The listing builds one solid part. Answer for the finished solid, in the listing's coordinates (mm). A direction names the side the tool comes from. Coordinates: 2 decimals unless noted, no trailing zeros. Loops run counter-clockwise (first coordinate to the right, second up) from the corner with the lowest first, then second, coordinate; pieces in that order, holes last. Notation, with made-up numbers: M 12,-7 L 57,-7 A13 cw 57,4 Z; hole C 51.5,86.5 d1. An arc over 180 degrees is marked long. Answer as a JSON object with one key per item and string values. Group by question number.
1. A cutting plane is placed at A-A on z = 5. Give the vertices of the cut face in (x, y).
2. A cutting plane is placed at C-C on y = 19.75. Give the vertices of the cut face in (x, z), and give its area (3 significant figures).
3. Given pin 1 (10 mm diameter, centred on x = -7, y = 18.5, fed in from +Z); pin 2 (5 mm diameter, centred on x = -9.5, y = 10, fed in from +Z), each flat-ended and moving along its own axis, determine where each tip first touches the part or whether it passes through.
4. Straight lines are drawn through the part: L1, parallel to X at y = 5, z = 4.5; L2, parallel to Y at x = -19, z = 6.75; L3, parallel to Z at x = -18.5, y = 19. For each, find the intervals that lie inside material, in ascending order.
5. Determine the mould class of faces 1 (the face through (2, 10, 8)), 2 (the face through (-10, 10, 3)), 3 (the face through (-10, 20.5, 9)), 4 (the face through (-10.4, -1.2, 0.7)) for opening direction Y: released by +Y, released by -Y, zero draft, split by the parting line, or undercut.
6. A cutting plane is placed at B-B on x = -4.75. Give the vertices of the cut face in (y, z), and give its area (3 significant figures).
7. For faces 5 (the face through (-22, 10, 1)), 6 (the face through (0.5, 10.1, 14.5)), determine the directions among +Z, -Z, +X, -X, +Y, -Y from which every point of the face is accessible in a straight line to the end or side of a thin tool.
from build123d import *

# Parameters (mm, degrees)
SKETCH_W        = 20.5
SKETCH_H        = 20.5
PAD_DEPTH       = 15
SKETCH001_W     = 24.5
SKETCH001_H     = 24.5
PAD001_DEPTH    = 15
PAD001_FACE7_W  = 20.5
PAD001_FACE7_H  = 20.5
POCKET_DEPTH    = 12
CHAMFER_SIZE    = 1
CHAMFER001_SIZE = 1.5


with BuildPart() as part:
    # Sketch → Pad (new body)
    with BuildSketch(Plane.XY):
        with Locations((-10.25, 10.25)):
            Rectangle(SKETCH_W, SKETCH_H)
    extrude(amount=PAD_DEPTH)

    # Sketch001 (on Face6 of Pad) → Pad001 (join)
    with BuildSketch(Plane.XY.offset(15)):
        with Locations((-10.25, 10.25)):
            Rectangle(SKETCH001_W, SKETCH001_H)
    extrude(amount=-PAD001_DEPTH)

    # Pad001 Face7 → Pocket (cut)
    with BuildSketch(Plane(origin=(-10.25, 10.25, 15), x_dir=(0, 1, 0), z_dir=(0, 0, 1))):
        Rectangle(PAD001_FACE7_W, PAD001_FACE7_H)
    extrude(amount=-POCKET_DEPTH, mode=Mode.SUBTRACT)

    # Chamfer
    chamfer_edges = [part.edges().sort_by_distance(p)[0] for p in [
        (-20.5, 10.25, 15),
        (-10.25, 20.5, 15),
        (0, 10.25, 15),
        (-10.25, 0, 15),
    ]]
    chamfer(chamfer_edges, length=CHAMFER_SIZE)

    # Chamfer001
    chamfer001_edges = [part.edges().sort_by_distance(p)[0] for p in [
        (-10.25, 22.5, 0),
        (-22.5, 10.25, 0),
        (-10.25, -2, 0),
        (2, 10.25, 0),
    ]]
    chamfer(chamfer001_edges, length=CHAMFER001_SIZE)


solid = part.part
From the geometry:
{
 "1": {"outline": "M -22.5,-2 L 2,-2 L 2,22.5 L -22.5,22.5 Z; hole M -20.5,0 L 0,0 L 0,20.5 L -20.5,20.5 Z"},
 "2": {"outline": "M -22.5,1.5 L -21,0 L 0.5,0 L 2,1.5 L 2,15 L 1,15 L 0,14 L 0,3 L -20.5,3 L -20.5,14 L -21.5,15 L -22.5,15 Z", "area": "118 mm²"},
 "3": {"pin 1": "stops at z = 15", "pin 2": "stops at z = 3"},
 "4": {"L1": "x = -22.5 to -20.5, 0 to 2", "L2": "y = -2 to 0, 20.5 to 22.5", "L3": "z = 0 to 3"},
 "5": {"face 1": "zero draft", "face 2": "undercut", "face 3": "undercut", "face 4": "released by -Y"},
 "6": {"outline": "M -2,1.5 L -0.5,0 L 21,0 L 22.5,1.5 L 22.5,15 L 21.5,15 L 20.5,14 L 20.5,3 L 0,3 L 0,14 L -1,15 L -2,15 Z", "area": "118 mm²"},
 "7": {"face 5": "-Z, -X, +Y, -Y", "face 6": "+Z"}
}
